Read the model definition and answer for the solid it produces. Units are mm, in the model's axes. A direction names the side the tool comes from. Give positions to 0.01 mm unless a question says otherwise; leave off trailing zeros. Order: outer loops, then holes, each group sorted by start corner. A loop starts at its lowest first (then second) coordinate and runs counter-clockwise, first axis right, second up. Notation, with made-up numbers: (-11, 33.5) -> (27, 33.5) arc R5 cw to (27, 39.5) -> close; hole circle Ø3 at (22, -33). An arc over 180 degrees is marked (long way). Use one line per item in the form item = value.
```python
from build123d import *

# Parameters (mm, degrees)
F0_R     = 2.15265
F1_DEPTH = 9.525
F2_R     = 2.15265
F3_DEPTH = 9.525
F4_R     = 2.15265
F5_DEPTH = 9.525


with BuildPart() as f1:
    # F0 (on Top) → F1 (new body)
    with BuildSketch(Plane.XY):
        Polygon((14.2875, 0), (0, 0), (0, 14.2875), (-9.525, 14.2875), (-9.525, 1.5875), (-12.7, 1.5875), (-12.7, -4.7625), (-9.525, -4.7625), (-9.525, -9.525), (-4.7625, -9.525), (-4.7625, -12.7), (1.5875, -12.7), (1.5875, -9.525), (14.2875, -9.525), align=None)
        with Locations((-4.7625, -4.7625)):
            Circle(F0_R, mode=Mode.SUBTRACT)
    extrude(amount=F1_DEPTH)

    # F2 (on face) → F3 (cut, through all)
    with BuildSketch(Plane(origin=(0, 0, 0), x_dir=(-1, 0, 0), z_dir=(0, 1, 0))):
        with Locations((-9.525, 4.7625)):
            Circle(F2_R)
    extrude(amount=-F3_DEPTH, mode=Mode.SUBTRACT)

    # F4 (on face) → F5 (cut, through all)
    with BuildSketch(Plane.YZ):
        with Locations((9.525, 4.7625)):
            Circle(F4_R)
    extrude(amount=-F5_DEPTH, mode=Mode.SUBTRACT)


solid = f1.part
```
Item 1: Which of the six approach directions +Z, -Z, +X, -X, +Y, -Y give full straight-line access (tool end or side, diameter ignored) to faces 4 (the flat face through (0, 7, 5)), 5 (the flat face through (-9.525, 7, 5)), 6 (the flat face through (-11, -4.762, 5)), 7 (the flat face through (6, -9.525, 5))?
Checks:
face_4 = +Z, -Z, +X, +Y
face_5 = +Z, -Z, -X, +Y
face_6 = +Z, -Z, -X, -Y
face_7 = +Z, -Z, +X, -Y
Item 2: Given pin 1 Ø3.5 at (y, z) = (-12, 4.5) entering from +X; pin 2 Ø5 at (x, z) = (9.52, 4.76) entering from +Y; pin 3 Ø5 at (y, z) = (-7.5, 3) entering from -X (3 decimals), each flat-ended and moving along its own axis, determine where each tip first touches the part or whether it passes through.
Checks:
pin_1 = 1.59
pin_2 = 0
pin_3 = -9.525
Item 3: The part is cut by section D-D on z = 8.75. Give the vertices of the cut face in (x, y) (1 decimal), and give its area (3 significant figures).
Checks:
outline = (-12.7, -4.8) -> (-9.5, -4.8) -> (-9.5, -9.5) -> (-4.8, -9.5) -> (-4.8, -12.7) -> (1.6, -12.7) -> (1.6, -9.5) -> (14.3, -9.5) -> (14.3, 0) -> (0, 0) -> (0, 14.3) -> (-9.5, 14.3) -> (-9.5, 1.6) -> (-12.7, 1.6) -> close; hole circle Ø4.3 at (-4.8, -4.8)
area = 389 mm²
Item 4: Determine the mould class of faces 1 (the cylindrical face through (-5.229, -6.864, 4.696)), 2 (the flat face through (-4.762, -11, 5)), 3 (the cylindrical face through (-4.7, 10.68, 6.58)) for opening direction X: +X half, -X half, draft (parallel to the pull), parting line (faces both ways), or undercut.
Checks:
face_1 = undercut
face_2 = -X half
face_3 = draft
Item 5: The part is cut by section C-C on y = 8.25. Give the vertices of the cut face in (x, z) (3 decimals), and give its area (3 significant figures).
Checks:
outline = (-9.525, 0) -> (0, 0) -> (0, 3.028) -> (-9.525, 3.028) -> close; (-9.525, 6.497) -> (0, 6.497) -> (0, 9.525) -> (-9.525, 9.525) -> close
area = 57.7 mm²
Item 6: Straight lines are drawn through the part: L1, parallel to Y at x = -5.5, z = 6.25 (1 decimal); L2, parallel to Y at x = 11, z = 7 (3 decimals); L3, parallel to X at y = 1.25, z = 2.5. For each, find the intervals that lie inside material, in ascending order. Write a range as from..to.
Checks:
L1 = -9.5..-6.8, -2.7..8, 11.1..14.3
L2 = -9.525..0
L3 = -12.7..0
Item 7: The part is cut by section B-B on y = -4. Give the vertices of the cut face in (x, z) (1 decimal).
Checks:
outline = (-12.7, 0) -> (-6.8, 0) -> (-6.8, 9.5) -> (-12.7, 9.5) -> close; (-2.7, 0) -> (14.3, 0) -> (14.3, 9.5) -> (-2.7, 9.5) -> close; hole circle Ø4.3 at (9.5, 4.8)
Item 8: The part is cut by section A-A on z = 6.5. Give the vertices of the cut face in (x, y) (1 decimal).
Checks:
outline = (-12.7, -4.8) -> (-9.5, -4.8) -> (-9.5, -9.5) -> (-4.8, -9.5) -> (-4.8, -12.7) -> (1.6, -12.7) -> (1.6, -9.5) -> (8.3, -9.5) -> (8.3, 0) -> (0, 0) -> (0, 8.3) -> (-9.5, 8.3) -> (-9.5, 1.6) -> (-12.7, 1.6) -> close; (-9.5, 10.8) -> (0, 10.8) -> (0, 14.3) -> (-9.5, 14.3) -> close; (10.8, -9.5) -> (14.3, -9.5) -> (14.3, 0) -> (10.8, 0) -> close; hole circle Ø4.3 at (-4.8, -4.8)
